Geometry check sheet. Reference: the model listing, model coordinates, mm. Face numbers are marked on the shaded views. A direction names the side the tool comes from. Round coordinates to 2 decimals unless told otherwise and drop trailing zeros. Loops run counter-clockwise (first coordinate to the right, second up) from the corner with the lowest first, then second, coordinate; pieces in that order, holes last. Notation, with made-up numbers: M -38,72.5 L -18,72.5 A6 ccw -18,83.5 Z; hole C 46.5,22 d1. An arc over 180 degrees is marked long. Answer in a Markdown table with one row per item. Add a question column.
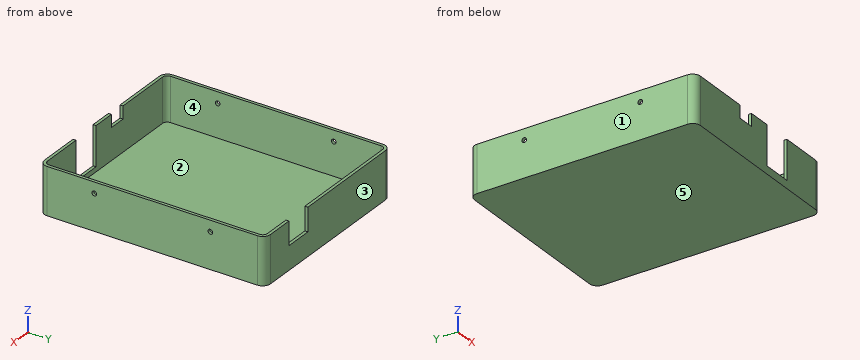
```python
from build123d import *

# Parameters (mm, degrees)
F0_W      = 119
F0_H      = 144
F1_DEPTH  = 30
F2_T      = -1.9
F3_R      = 5
F4_R      = 3
F5_R      = 1.5
F6_DEPTH  = 119.001
F7_W      = 19
F7_H      = 25
F7_W_2    = 11
F7_H_2    = 8
F8_DEPTH  = 3
F9_W      = 18
F9_H      = 15
F10_DEPTH = 3


with BuildPart() as f1:
    # F0 (on Top) → F1 (new body)
    with BuildSketch(Plane.XY):
        Rectangle(F0_W, F0_H)
    extrude(amount=F1_DEPTH)

    # F2
    f2_openings = [f1.faces().sort_by_distance(p)[0] for p in [
        (0, 0, 30),
    ]]
    offset(amount=F2_T, openings=f2_openings)

    # F3
    f3_edges = [f1.edges().sort_by_distance(p)[0] for p in [
        (-59.5, -72, 15),
        (59.5, -72, 15),
        (59.5, 72, 15),
        (-59.5, 72, 15),
    ]]
    fillet(f3_edges, radius=F3_R)

    # F4
    f4_edges = [f1.edges().sort_by_distance(p)[0] for p in [
        (-57.6, -70.1, 15.95),
        (57.6, -70.1, 15.95),
        (-57.6, 70.1, 15.95),
        (57.6, 70.1, 15.95),
    ]]
    fillet(f4_edges, radius=F4_R)

    # F5 (on face) → F6 (cut, through all)
    with BuildSketch(Plane(origin=(-59.5, 0, 0), x_dir=(0, -1, 0), z_dir=(-1, 0, 0))):
        with Locations((-37, 23)):
            Circle(F5_R)
        with Locations((37, 23)):
            Circle(F5_R)
    extrude(amount=-F6_DEPTH, mode=Mode.SUBTRACT)

    # F7 (on face) → F8 (cut)
    with BuildSketch(Plane.XZ.offset(72)):
        with Locations((18, 17.5)):
            Rectangle(F7_W, F7_H)
        with Locations((-11.5, 26)):
            Rectangle(F7_W_2, F7_H_2)
    extrude(amount=-F8_DEPTH, mode=Mode.SUBTRACT)

    # F9 (on face) → F10 (cut)
    with BuildSketch(Plane(origin=(0, 72, 0), x_dir=(-1, 0, 0), z_dir=(0, 1, 0))):
        with Locations((-28, 22.5)):
            Rectangle(F9_W, F9_H)
    extrude(amount=-F10_DEPTH, mode=Mode.SUBTRACT)


solid = f1.part
```
1) Cross-section at C-C, the plane y = 49. Record the boundary of the cut face in (x, z).
2) Thickness scan on L1, parallel to Y at x = -31.5, z = 19; L2, parallel to X at y = 58.5, z = 23.75; L3, parallel to Z at x = 59.1, y = 37. Record the ranges inside material, lowest first. Write a range as [from, to].
3) Set-up check for the marked faces 4 and 5: record each of +Z, -Z, +X, -X, +Y, -Y from which the full face is reachable in a straight line by a thin tool's end or side.
4) Cross-section at B-B, the plane x = -11. Record the boundary of the cut face in (y, z), plus the area to 3 significant figures.
5) Draft check along X on the marked faces 1, 2 and 3. Enter one of: +X half, -X half, draft (parallel to the pull), parting line (faces both ways), or undercut.
6) Cross-section at A-A, the plane z = 27. Record the boundary of the cut face in (x, y), plus the area to 3 significant figures.
7) Go/stop test with flat-tipped pins: pin 1 (1 mm diameter, centred on y = -70.5, z = 11.5, fed in from +X); pin 2 (1 mm diameter, centred on x = -9.5, y = -70.5, fed in from +Z); pin 3 (1 mm diameter, centred on y = -71, z = 28, fed in from -X). Record where each tip stops, or that it passes through.
Worked answers:
| question | item | result |
|---|---|---|
| 1 | outline | M -59.5,0 L 59.5,0 L 59.5,30 L 57.6,30 L 57.6,1.9 L -57.6,1.9 L -57.6,30 L -59.5,30 Z |
| 2 | L1 | y = [-72, -70.1], [70.1, 72] |
| 2 | L2 | x = [-59.5, -57.6], [57.6, 59.5] |
| 2 | L3 | z = [0, 21.5], [24.5, 30] |
| 3 | face 4 | +Z |
| 3 | face 5 | -Z, +X, -X, +Y, -Y |
| 4 | outline | M -72,0 L 72,0 L 72,30 L 70.1,30 L 70.1,1.9 L -70.1,1.9 L -70.1,22 L -72,22 Z |
| 4 | area | 365 mm2 |
| 5 | face 1 | -X half |
| 5 | face 2 | undercut |
| 5 | face 3 | draft |
| 6 | outline | M -59.5,-67 A5 ccw -54.5,-72 L -17,-72 L -17,-70.1 L -54.6,-70.1 A3 cw -57.6,-67.1 L -57.6,67.1 A3 cw -54.6,70.1 L 19,70.1 L 19,72 L -54.5,72 A5 ccw -59.5,67 Z; M -6,-72 L 8.5,-72 L 8.5,-70.1 L -6,-70.1 Z; M 27.5,-72 L 54.5,-72 A5 ccw 59.5,-67 L 59.5,67 A5 ccw 54.5,72 L 37,72 L 37,70.1 L 54.6,70.1 A3 cw 57.6,67.1 L 57.6,-67.1 A3 cw 54.6,-70.1 L 27.5,-70.1 Z |
| 6 | area | 880 mm2 |
| 7 | pin 1 | stops at x = 58.5 |
| 7 | pin 2 | stops at z = 22 |
| 7 | pin 3 | stops at x = -58.07 |
